Design review of the part built by this model. Coordinates are the model's own, in mm. A direction names the side the tool comes from. Give positions to 0.01 mm unless a question says otherwise; leave off trailing zeros. Loops run counter-clockwise (first coordinate to the right, second up) from the corner with the lowest first, then second, coordinate; pieces in that order, holes last. Notation, with made-up numbers: (-34, -32) -> (-10, -32) arc R22 cw to (-10, -18) -> close; hole circle Ø4 at (67, 84). An arc over 180 degrees is marked (long way). Use CSV: the item, a comma, the result in double quotes. Start each with the question number.
Item 1: For faces 4 (the face through (-108, 0, -8)), 5 (the face through (-103.3, -4.2, -2.5)), 6 (the face through (-103, -4.7, -1)), list the 3-axis set-ups (+Z, -Z, +X, -X, +Y, -Y) from which the entire face can be reached by the end or side of a thin tool; tool diameter is ignored.
Item 2: We need section A-A (z = -4.5). State the section outline as (x, y) points.
Item 3: We need section C-C (y = -12). State the section outline as (x, z) points, plus the area to 3 significant figures.
Item 4: We need section D-D (x = -101). State the section outline as (y, z) points, plus the area to 3 significant figures.
Item 5: The part is to be moulded in two halves that separate along Y. For faces 1 (the face through (-108, -15, -7)), 2 (the face through (-103, -4.7, -4)), 3 (the face through (-109, 12, -2)), say which applies: +Y half, -Y half, draft (parallel to the pull), parting line (faces both ways), or undercut.
Item 6: Wall thickness on line 1 along Y through (x, z) = (-106, -3.25); line 2 along Y through (x, z) = (-109, -0.75); line 3 along Z through (x, y) = (-99, 2.5): over which ranges is each line inside the solid? List them lowest first. Write a range as from..to.
Item 7: We need section B-B (x = -120). State the section outline as (y, z) points, plus the area to 3 significant figures.
Item 8: Clearance check with flat-ended pins moving along their axes: pin 1 (0.6 mm diameter, centred on x = -105.5, z = -1, fed in from -Y); pin 2 (3 mm diameter, centred on y = 0, z = -1, fed in from +X); pin 3 (4.5 mm diameter, centred on x = -100, y = 0.5, fed in from +Z). State where each tip first meets the part, or that it passes through.
from build123d import *

# Parameters (mm, degrees)
F0_W      = 16
F0_H      = 6
F1_DEPTH  = 95
F2_DEPTH  = 5
F3_R      = 2
F4_DEPTH  = 127.001
F5_SIZE   = 0.49999
F6_DEPTH  = 25
F8_DEPTH  = 25
F9_W      = 318.6057507992
F9_H      = 243.2989366353
F10_DEPTH = 19.501
F12_DEPTH = 10
F14_DEPTH = 8.001
F15_SIZE  = 5
F16_SIZE  = 5


# Not quite as in the source:
# - a fillet or chamfer is up to 0.001 mm smaller than in the source, because OpenCascade refuses the exact size


with BuildPart() as f1:
    # F0 (on Top) → F1 (new body)
    with BuildSketch(Plane.XY):
        Polygon((-8, -4.5), (63.5, -4.5), (63.5, 4.5), (-26, 4.5), (-28, 4.5), (-44, 4.5), (-46, 4.5), (-63.5, 4.5), (-63.5, -4.5), (-28, -4.5), (-26, -4.5), (-10, -4.5), align=None)
        with Locations((-54, 0)):
            Rectangle(F0_W, F0_H, mode=Mode.SUBTRACT)
        with Locations((-36, 0)):
            Rectangle(F0_W, F0_H, mode=Mode.SUBTRACT)
        with Locations((-18, 0)):
            Rectangle(F0_W, F0_H, mode=Mode.SUBTRACT)
        Rectangle(F0_W, F0_H, mode=Mode.SUBTRACT)
        with Locations((18, 0)):
            Rectangle(F0_W, F0_H, mode=Mode.SUBTRACT)
        with Locations((36, 0)):
            Rectangle(F0_W, F0_H, mode=Mode.SUBTRACT)
        with Locations((54, 0)):
            Rectangle(F0_W, F0_H, mode=Mode.SUBTRACT)
    extrude(amount=F1_DEPTH)

    # F0 (on Top) → F2 (join)
    with BuildSketch(Plane.XY):
        Polygon((-8, -4.5), (63.5, -4.5), (63.5, 4.5), (-26, 4.5), (-28, 4.5), (-44, 4.5), (-46, 4.5), (-63.5, 4.5), (-63.5, -4.5), (-28, -4.5), (-26, -4.5), (-10, -4.5), align=None)
        with Locations((-54, 0)):
            Rectangle(F0_W, F0_H, mode=Mode.SUBTRACT)
        with Locations((-36, 0)):
            Rectangle(F0_W, F0_H, mode=Mode.SUBTRACT)
        with Locations((-18, 0)):
            Rectangle(F0_W, F0_H, mode=Mode.SUBTRACT)
        Rectangle(F0_W, F0_H, mode=Mode.SUBTRACT)
        with Locations((18, 0)):
            Rectangle(F0_W, F0_H, mode=Mode.SUBTRACT)
        with Locations((36, 0)):
            Rectangle(F0_W, F0_H, mode=Mode.SUBTRACT)
        with Locations((54, 0)):
            Rectangle(F0_W, F0_H, mode=Mode.SUBTRACT)
        with Locations((-54, 0)):
            Rectangle(F0_W, F0_H)
        with Locations((-36, 0)):
            Rectangle(F0_W, F0_H)
        with Locations((-18, 0)):
            Rectangle(F0_W, F0_H)
        Rectangle(F0_W, F0_H)
        with Locations((18, 0)):
            Rectangle(F0_W, F0_H)
        with Locations((36, 0)):
            Rectangle(F0_W, F0_H)
        with Locations((54, 0)):
            Rectangle(F0_W, F0_H)
    extrude(amount=-F2_DEPTH)

    # F3 (on face) → F4 (cut, through all)
    with BuildSketch(Plane(origin=(-63.5, 0, 0), x_dir=(0, -1, 0), z_dir=(-1, 0, 0))):
        with Locations((-6, -2.5)):
            Circle(F3_R)
        with Locations((6, -2.5)):
            Circle(F3_R)
    extrude(amount=-F4_DEPTH, mode=Mode.SUBTRACT)

    # F5 (size 0.5 in the source; OpenCascade refuses exactly that, so slightly less here)
    f5_edges = [f1.edges().sort_by_distance(p)[0] for p in [
        (-63.5, 4.5, 46.911438),
        (-63.5, -4.5, 46.911438),
        (0, 4.5, -5),
        (-63.5, 0, -5),
        (-63.5, 4, -2.5),
        (0, 4.5, 95),
        (-63.5, 0, 95),
        (0, -4.5, 95),
        (63.5, 0, 95),
        (63.5, 0, -5),
        (63.5, 4.5, 46.911438),
        (63.5, -4.5, 46.911438),
        (-63.5, -4, -2.5),
        (63.5, 4, -2.5),
        (63.5, -4, -2.5),
        (54, -3, 95),
        (46, 0, 95),
        (54, 3, 95),
        (62, 0, 95),
        (44, 0, 95),
        (36, 3, 95),
        (36, -3, 95),
        (8, 0, 95),
        (10, 0, 95),
        (18, 3, 95),
        (18, -3, 95),
        (26, 0, 95),
        (28, 0, 95),
        (0, 3, 95),
        (0, -3, 95),
        (-8, 0, 95),
        (-10, 0, 95),
        (-18, -3, 95),
        (-26, 0, 95),
        (-18, 3, 95),
        (-36, 3, 95),
        (-28, 0, 95),
        (-36, -3, 95),
        (-54, 3, 95),
        (-62, 0, 95),
        (-54, -3, 95),
        (-46, 0, 95),
        (-44, 0, 95),
    ]]
    chamfer(f5_edges, length=F5_SIZE)

    # F3 (on face) → F6 (join)
    with BuildSketch(Plane(origin=(-63.5, 0, 0), x_dir=(0, -1, 0), z_dir=(-1, 0, 0))):
        with BuildLine():
            ThreePointArc((-4.5, -1.1771243445), (-4.1291713066, -1.7928932188), (-4, -2.5))
            ThreePointArc((-4, -2.5), (-4.1291713066, -3.2071067812), (-4.5, -3.8228756555))
            Line((-4.5, -3.8228756555), (-4.5, -5))
            Line((-4.5, -5), (4.5, -5))
            Line((4.5, -5), (4.5, -3.8228756555))
            ThreePointArc((4.5, -3.8228756555), (4, -2.5), (4.5, -1.1771243445))
            Line((4.5, -1.1771243445), (4.5, 95))
            Line((4.5, 95), (-4.5, 95))
            Line((-4.5, 95), (-4.5, -1.1771243445))
        make_face()
    extrude(amount=F6_DEPTH)


with BuildPart() as f8:
    # F7 (on face) → F8 (new body)
    with BuildSketch(Plane(origin=(-88.5, 0, 0), x_dir=(0, -1, 0), z_dir=(-1, 0, 0))):
        with BuildLine():
            Line((15, 0), (4.7, 0))
            Line((4.7, 0), (4.7, -1.2550100402))
            ThreePointArc((4.7, -1.2550100402), (4.2, -2.5), (4.7, -3.7449899598))
            Line((4.7, -3.7449899598), (4.7, -5.2))
            Line((4.7, -5.2), (-4.7, -5.2))
            Line((-4.7, -5.2), (-4.7, -3.7449899598))
            ThreePointArc((-4.7, -3.7449899598), (-4.2, -2.5), (-4.7, -1.2550100402))
            Line((-4.7, -1.2550100402), (-4.7, 0))
            Line((-4.7, 0), (-15, 0))
            Line((-15, 0), (-15, -8))
            Line((-15, -8), (15, -8))
            Line((15, -8), (15, 0))
        make_face()
    extrude(amount=F8_DEPTH)


with BuildPart() as f10_tool:
    # F9 (on face) → F10 (new body, through all)
    with BuildSketch(Plane(origin=(0, 4.5, 0), x_dir=(-1, 0, 0), z_dir=(0, 1, 0))):
        with Locations((-68.3380588889, 100.3342196345)):
            Rectangle(F9_W, F9_H)
    extrude(amount=-F10_DEPTH)


with BuildPart() as f1_1:
    add(f1.part)

    # F10: cut by f10_tool
    add(f10_tool.part, mode=Mode.SUBTRACT)


with BuildPart() as f8_1:
    add(f8.part)

    # F10: cut by f10_tool
    add(f10_tool.part, mode=Mode.SUBTRACT)

    # F11 (on face) → F12 (join)
    with BuildSketch(Plane(origin=(-113.5, 0, 0), x_dir=(0, -1, 0), z_dir=(-1, 0, 0))):
        with BuildLine():
            Line((-4.7, -1.2550100402), (-4.7, 0))
            Line((-4.7, 0), (-15, 0))
            Line((-15, 0), (-15, -8))
            Line((-15, -8), (15, -8))
            Line((15, -8), (15, 0))
            Line((15, 0), (4.7, 0))
            Line((4.7, 0), (4.7, -1.2550100402))
            ThreePointArc((4.7, -1.2550100402), (4.2, -2.5), (4.7, -3.7449899598))
            Line((4.7, -3.7449899598), (4.7, -5.2))
            Line((4.7, -5.2), (-4.7, -5.2))
            Line((-4.7, -5.2), (-4.7, -3.7449899598))
            ThreePointArc((-4.7, -3.7449899598), (-4.2, -2.5), (-4.7, -1.2550100402))
        make_face()
        with BuildLine():
            Line((4.7, 0), (-4.7, 0))
            Line((-4.7, 0), (-4.7, -1.2550100402))
            ThreePointArc((-4.7, -1.2550100402), (-4.2, -2.5), (-4.7, -3.7449899598))
            Line((-4.7, -3.7449899598), (-4.7, -5.2))
            Line((-4.7, -5.2), (4.7, -5.2))
            Line((4.7, -5.2), (4.7, -3.7449899598))
            ThreePointArc((4.7, -3.7449899598), (4.2, -2.5), (4.7, -1.2550100402))
            Line((4.7, -1.2550100402), (4.7, 0))
        make_face()
    extrude(amount=F12_DEPTH)

    # F13 (on face) → F14 (cut, through all)
    with BuildSketch(Plane(origin=(0, 0, -8), x_dir=(1, 0, 0), z_dir=(0, 0, -1))):
        Polygon((-93.395665288, -19.6107532829), (-75.3739327192, -19.6107532829), (-75.3739327192, 58.0060165375), (-93.395665288, 58.0060165375), (-93.395665288, 15), (-90.9648165107, 15), (-90.9648165107, -4.5), (-88.5, -4.5), (-88.5, -15), (-93.395665288, -15), align=None)
        Polygon((-93.395665288, 15), (-93.395665288, -15), (-88.5, -15), (-88.5, -4.5), (-90.9648165107, -4.5), (-90.9648165107, 15), align=None)
    extrude(amount=-F14_DEPTH, mode=Mode.SUBTRACT)

    # F15
    f15_edges = [f8_1.edges().sort_by_distance(p)[0] for p in [
        (-108.447833, 15, 0),
        (-108.447833, -15, 0),
    ]]
    chamfer(f15_edges, length=F15_SIZE)

    # F16
    f16_edges = [f8_1.edges().sort_by_distance(p)[0] for p in [
        (-123.5, 0, 0),
    ]]
    chamfer(f16_edges, length=F16_SIZE)


solid = f8_1.part
Results found:
1,face 4,"-Z, +X, -X, +Y, -Y"
1,face 5,"+X"
1,face 6,"+Z, +X"
2,outline,"(-123, -14.5) -> (-93.4, -14.5) -> (-93.4, -4.7) -> (-113.5, -4.7) -> (-113.5, 4.7) -> (-93.4, 4.7) -> (-93.4, 14.5) -> (-123, 14.5) -> close"
3,outline,"(-123.5, -8) -> (-93.4, -8) -> (-93.4, -2) -> (-120.5, -2) -> (-123.5, -5) -> close"
3,area,"176 mm²"
4,outline,"(-15, -8) -> (15, -8) -> (15, -5) -> (10, 0) -> (4.7, 0) -> (4.7, -1.26) arc R1.8 ccw to (4.7, -3.74) -> (4.7, -5.2) -> (-4.7, -5.2) -> (-4.7, -3.74) arc R1.8 ccw to (-4.7, -1.26) -> (-4.7, 0) -> (-10, 0) -> (-15, -5) -> close"
4,area,"168 mm²"
5,face 1,"-Y half"
5,face 2,"undercut"
5,face 3,"+Y half"
6,line 1,"-13.25..-4.36, 4.36..13.25"
6,line 2,"-10.75..-4.7, 4.7..10.75"
6,line 3,"-8..-5.2"
7,outline,"(-15, -8) -> (15, -8) -> (15, -5) -> (11.5, -1.5) -> (-11.5, -1.5) -> (-15, -5) -> close"
7,area,"183 mm²"
8,pin 1,"y = -11.3"
8,pin 2,"x = -113.5"
8,pin 3,"z = -5.2"
